The listing builds one solid part. Answer for the finished solid, in the listing's coordinates (mm). A direction names the side the tool comes from. Coordinates: 2 decimals unless noted, no trailing zeros. Write each loop counter-clockwise with the first axis right and the second up, starting at its lowest first coordinate (ties: lowest second). Pieces come first, ordered by that corner, then holes.
from build123d import *

# Parameters (mm, degrees)
SKETCH_3_W          = 43
SKETCH_3_H          = 49
EXTRUDE_2_DEPTH     = 3
SKETCH_6_R          = 11.1
SKETCH_6_R_2        = 1.6
CUT_EXTRUDE_2_DEPTH = 45
SKETCH_7_W          = 43
SKETCH_7_H          = 3
EXTRUDE_4_DEPTH     = 52
SKETCH_8_R          = 1.6
SKETCH_8_R_2        = 1.55
CUT_EXTRUDE_3_DEPTH = 45
FILLET_1_R          = 5


with BuildPart() as part:
    # 草图3 → 凸台-拉伸2 (new body)
    with BuildSketch(Plane.XY):
        with Locations((21.5, -24.5)):
            Rectangle(SKETCH_3_W, SKETCH_3_H)
    extrude(amount=EXTRUDE_2_DEPTH)

    # 草图6 → 切除-拉伸2 (cut)
    with BuildSketch(Plane(origin=(0, 0, 0), x_dir=(-1, 0, 0), z_dir=(0, 0, -1))):
        with Locations((-21.5, -21.15)):
            Circle(SKETCH_6_R)
        with Locations((-37, -5.65)):
            Circle(SKETCH_6_R_2)
        with Locations((-6, -5.65)):
            Circle(SKETCH_6_R_2)
        with Locations((-6, -36.65)):
            Circle(SKETCH_6_R_2)
        with Locations((-37, -36.65)):
            Circle(SKETCH_6_R_2)
    extrude(amount=-CUT_EXTRUDE_2_DEPTH, mode=Mode.SUBTRACT)

    # 草图7 → 凸台-拉伸4 (add)
    with BuildSketch(Plane(origin=(0, 0, 0), x_dir=(-1, 0, 0), z_dir=(0, 0, -1))):
        with Locations((-21.5, -47.5)):
            Rectangle(SKETCH_7_W, SKETCH_7_H)
    extrude(amount=EXTRUDE_4_DEPTH)

    # 草图8 → 切除-拉伸3 (cut)
    with BuildSketch(Plane(origin=(0, -46, 0), x_dir=(1, 0, 0), z_dir=(0, 1, 0))):
        with Locations((11, 10.65)):
            Circle(SKETCH_8_R)
        with Locations((11, 22.65)):
            Circle(SKETCH_8_R)
        with Locations((32, 10.65)):
            Circle(SKETCH_8_R)
        with Locations((32, 22.65)):
            Circle(SKETCH_8_R)
        with Locations((21.5, 44)):
            Circle(SKETCH_8_R_2)
    extrude(amount=-CUT_EXTRUDE_3_DEPTH, mode=Mode.SUBTRACT)

    # 圆角1
    fillet_1_edges = [part.edges().sort_by_distance(p)[0] for p in [
        (43, -47.5, -52),
        (0, -47.5, -52),
        (0, 0, 1.5),
        (43, 0, 1.5),
    ]]
    fillet(fillet_1_edges, radius=FILLET_1_R)


solid = part.part
Q1. The part is cut by section A-A, the plane z = -44. Write down the section's boundary in (x, y).
Answers below:
outline: (0, -49) - (19.95, -49) - (19.95, -46) - (0, -46) - close; (23.05, -49) - (43, -49) - (43, -46) - (23.05, -46) - close
Q2. The part is cut by section B-B, the plane y = -21.15. Write down the section's boundary in (x, z), then the cut area to 3 significant figures.
Answers below:
outline: (0, 0) - (10.4, 0) - (10.4, 3) - (0, 3) - close; (32.6, 0) - (43, 0) - (43, 3) - (32.6, 3) - close
area: 62.4 mm2
Q3. Given pin 1 (10 mm diameter, centred on x = 11, y = -37, fed in from -Z); pin 2 (4 mm diameter, centred on x = 11, z = -22.65, fed in from +Y), each flat-ended and moving along its own axis, determine where each tip first touches the part or whether it passes through.
Answers below:
pin 1: stops at z = 0
pin 2: stops at y = -46
Q4. Find the intervals of material crossed by probe 1 along X at (y, z) = (-47.4, -22.65); probe 2 along Z at (x, y) = (21.5, -47.15); probe 3 along Y at (x, z) = (27, -5.5), in increasing order.
Answers below:
probe 1: x = 0 to 9.4, 12.6 to 30.4, 33.6 to 43
probe 2: z = -52 to -45.55, -42.45 to 3
probe 3: y = -49 to -46
Q5. Determine the mould class of faces 1 (the face through (2, -1, 2)), 2 (the face through (22, -47, -52)), 3 (the face through (9.4, -47.5, -10.7)) for opening direction X: released by +X, released by -X, zero draft, split by the parting line, or undercut.
Answers below:
face 1: released by -X
face 2: zero draft
face 3: undercut
Q6. The part is cut by section C-C, the plane x = 21.5. Write down the section's boundary in (y, z), then the cut area to 3 significant figures.
Answers below:
outline: (-49, -52) - (-46, -52) - (-46, -45.55) - (-49, -45.55) - close; (-49, -42.45) - (-46, -42.45) - (-46, 0) - (-32.25, 0) - (-32.25, 3) - (-49, 3) - close; (-10.05, 0) - (0, 0) - (0, 3) - (-10.05, 3) - close
area: 227 mm2
Q7. The part is cut by section D-D, the plane z = -10.65. Write down the section's boundary in (x, y).
Answers below:
outline: (0, -49) - (9.4, -49) - (9.4, -46) - (0, -46) - close; (12.6, -49) - (30.4, -49) - (30.4, -46) - (12.6, -46) - close; (33.6, -49) - (43, -49) - (43, -46) - (33.6, -46) - close
Q8. Which of the six approach directions +Z, -Z, +X, -X, +Y, -Y give full straight-line access (tool end or side, diameter ignored) to faces 4 (the face through (30.73, -47.48, -21.68)), 5 (the face through (22, -46, -26))?
Answers below:
face 4: +Y, -Y
face 5: -Z, +X, -X, +Y
